Here's how the part is built. I have some questions about the finished solid (model axes, mm). A direction names the side the tool comes from. Round coordinates to 2 decimals unless told otherwise and drop trailing zeros. Loops run counter-clockwise (first coordinate to the right, second up) from the corner with the lowest first, then second, coordinate; pieces in that order, holes last. Notation, with made-up numbers: (40, 32) - (45, 32) arc R19 cw to (45, 60) - close; hole circle Ø5 at (36.25, -31). An arc over 180 degrees is marked (long way). Answer as a JSON object with one key per item and string values. Group by question number.
1) I want a section at B-B, the plane z = 7.5. Please give me the cut outline in (x, y), then the cut area to 3 significant figures.
2) If I drill on line 1 along X through (y, z) = (69, -3); line 2 along Y through (x, z) = (13, 10.5); line 3 along Z through (x, y) = (8.5, 33.5), over which ranges is the centre line in solid material (lowest first)? Write a range as [from, to].
3) Will these pins go through, and if not, where does the flat tip stop? P1, Ø10, axis at x = 9, y = 21, coming from the +Z side; P2, Ø1.5, axis at y = 65, z = 2.5, coming from the +X side; P3, Ø7.5, axis at y = 33, z = 4.5, coming from the -X side.
4) Which directions (+Z, -Z, +X, -X, +Y, -Y) give clear straight access to the entire face, cutting with the end or side of a thin tool? Please do faces 1 (the face through (0, 45, 3)), 2 (the face through (12.7, 45, 3)), 3 (the face through (6, 54.853, -5)).
5) I want a section at A-A, the plane x = 5. Please give me the cut outline in (y, z) (3 decimals), then the cut area to 3 significant figures.
6) I want a section at C-C, the plane y = 45.5. Please give me the cut outline in (x, z).
7) I want a section at D-D, the plane x = 19. Please give me the cut outline in (y, z) (3 decimals), then the cut area to 3 significant figures.
from build123d import *

# Parameters (mm, degrees)
F0_W          = 12.7
F0_H          = 76.2
F1_DEPTH      = 6.35
F2_W          = 6.35
F2_H          = 25.4
F3_DEPTH      = 12.7
F3_DEPTH_BACK = 25.4
F4_W          = 12.7
F4_H          = 17.9375
F5_DEPTH      = 9.525
F5_DEPTH_BACK = 15.875


with BuildPart() as f1:
    # F0 (on Top) → F1 (new body)
    with BuildSketch(Plane.XY):
        with Locations((6.35, 41.040604)):
            Rectangle(F0_W, F0_H)
    extrude(amount=F1_DEPTH)

    # F2 (on face) → F3 (join, two sides)
    with BuildSketch(Plane(origin=(0, 0, 0), x_dir=(0, -1, 0), z_dir=(-1, 0, 0))) as f3_sk:
        with Locations((-75.965604, 3.175)):
            Rectangle(F2_W, F2_H)
    extrude(amount=F3_DEPTH)
    extrude(f3_sk.sketch, amount=-F3_DEPTH_BACK)

    # F4 (on face) → F5 (join, two sides)
    with BuildSketch(Plane.XY.offset(6.35)) as f5_sk:
        with Locations((6.35, 63.821854)):
            Rectangle(F4_W, F4_H)
    extrude(amount=F5_DEPTH)
    extrude(f5_sk.sketch, amount=-F5_DEPTH_BACK)


solid = f1.part
Outcome:
{
 "1": {"outline": "(-12.7, 72.79) - (0, 72.79) - (0, 54.85) - (12.7, 54.85) - (12.7, 72.79) - (25.4, 72.79) - (25.4, 79.14) - (-12.7, 79.14) - close", "area": "470 mm^2"},
 "2": {"line 1": "[0, 12.7]", "line 2": "[72.79, 79.14]", "line 3": "[0, 6.35]"},
 "3": {"P1": "z = 6.35", "P2": "x = 12.7", "P3": "x = 0"},
 "4": {"face 1": "+Z, -Z, -X, -Y", "face 2": "+Z, -Z, +X, -Y", "face 3": "-Z, +X, -X, -Y"},
 "5": {"outline": "(2.941, 0) - (54.853, 0) - (54.853, -9.525) - (79.141, -9.525) - (79.141, 15.875) - (54.853, 15.875) - (54.853, 6.35) - (2.941, 6.35) - close", "area": "947 mm^2"},
 "6": {"outline": "(0, 0) - (12.7, 0) - (12.7, 6.35) - (0, 6.35) - close"},
 "7": {"outline": "(72.791, -9.525) - (79.141, -9.525) - (79.141, 15.875) - (72.791, 15.875) - close", "area": "161 mm^2"}
}
